Autodesk Inventor part; units mm, degrees
ref_plane "YZ Plane" through (0, 0, 0) normal (1, 0, 0) x (0, 1, 0)
ref_plane "XZ Plane" through (0, 0, 0) normal (0, 1, 0) x (-1, 0, 0)
ref_plane "XY Plane" through (0, 0, 0) normal (0, 0, 1) x (1, 0, 0)
sketch "Sketch1" plane through (0, 0, 0) normal (0, 0, 1) x (1, 0, 0)
  line L0 (0, 38.1) -> (-2438.4, 38.1)
  line L1 (0, 1149.35) -> (0, -1111.25)
  line L2 (0, 0) -> (-2438.4, 0)
  line L3 (-2438.4, 1149.35) -> (-2438.4, -1111.25)
  line L4 (0, 1149.35) -> (-2438.4, 1149.35)
  line L5 (0, 86.9483) -> (-2331.2129, 1149.35)
  line L6 (-2438.4, 1100.5017) -> (-107.1871, 38.1)
  line L7 (-2331.2129, 1149.35) -> (-2438.4, 1149.35)
  line L8 (-2438.4, 1100.5017) -> (-2438.4, 1149.35)
  line L9 (0, 86.9483) -> (0, 38.1)
  line L10 (-107.1871, 38.1) -> (0, 38.1)
extrude "Extrusion1" add sketch "Sketch1" against normal blind 38.1 contours L0 L6 L3 L4 L5 L1
properties part number "s48x2x4b"
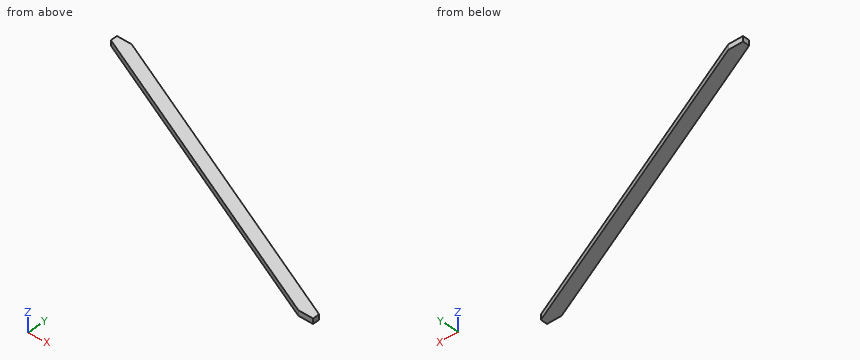
Can you work these out from the model? Positions are in its coordinate system, mm. Give positions to 0.01 mm unless a question says otherwise; leave off trailing zeros. Loops run counter-clockwise (first coordinate to the right, second up) from the corner with the lowest first, then second, coordinate; pieces in that order, holes last. Notation, with made-up numbers: M 11,-9.75 L 60,-9.75 A28 ccw 60,21.25 Z; hole C 19.25,-11.5 d11. An arc over 180 degrees is marked long. One line per item, written item: value. Start each with the question number.
1) If we section it at B-B, the plane x = -1701: Write out the boundary of the cut face in (y, z).
2) If we section it at C-C, the plane y = 471.5: Write out the boundary of the cut face in (x, z), and give its area (3 significant figures).
3) If we section it at A-A, the plane z = -26.5: Write out the boundary of the cut face in (x, y), and give its area (3 significant figures).
4) I'm going to push flat-ended pins straight in: pin 1 (12 mm diameter, centred on y = 931.5, z = -14.5, fed in from -X); pin 2 (6 mm diameter, centred on x = -322.5, z = -9, fed in from +Y); pin 3 (1.5 mm diameter, centred on y = 790, z = -9, fed in from -X). Where does each tip first touch, or does it pass through?
5) If I drill on line 1 (X direction, y = 312, z = -34.5); line 2 (X direction, y = 112, z = -24.5); line 3 (Y direction, x = -2023, z = -5.5), over which ranges is the centre line in solid material (lowest first)? Write a range as [from, to].
Completed:
1. outline: M 764.45,-38.1 L 862.14,-38.1 L 862.14,0 L 764.45,0 Z
2. outline: M -1058.19,-38.1 L -843.82,-38.1 L -843.82,0 L -1058.19,0 Z
2. area: 8,170 mm^2
3. outline: M -2438.4,1100.5 L -107.19,38.1 L 0,38.1 L 0,86.95 L -2331.21,1149.35 L -2438.4,1149.35 Z
3. area: 233,000 mm^2
4. pin 1: stops at x = -2080.73
4. pin 2: stops at y = 235.29
4. pin 3: stops at x = -1758.72
5. line 1: x = [-708.2, -493.83]
5. line 2: x = [-269.34, -54.97]
5. line 3: y = [911.19, 1008.89]
